from build123d import *

# Parameters (mm, degrees)
EXTRUDE_1_DEPTH     = 40
SKETCH_2_R          = 2
SKETCH_2_R_2        = 1.5
CUT_EXTRUDE_1_DEPTH = 112.803398875


with BuildPart() as part:
    # Эскиз1 → Бобышка-Вытянуть1 (new body)
    with BuildSketch(Plane.XY):
        with BuildLine():
            Line((0, 0), (100, 0))
            Line((100, 0), (100, 14))
            Line((100, 14), (84.933034374, 14))
            ThreePointArc((84.933034374, 14), (70, 15), (84.933034374, 16))
            Line((84.933034374, 16), (100, 16))
            Line((100, 16), (100, 30))
            Line((100, 30), (0, 30))
            Line((0, 30), (0, 16))
            Line((0, 16), (15.066965626, 16))
            ThreePointArc((15.066965626, 16), (30, 15), (15.066965626, 14))
            Line((15.066965626, 14), (0, 14))
            Line((0, 14), (0, 0))
        make_face()
    extrude(amount=EXTRUDE_1_DEPTH)

    # Эскиз2 → Вырез-Вытянуть1 (cut, through all)
    with BuildSketch(Plane.XZ):
        with Locations(Location((7.5, 30, 0), (0, 0, 270))):
            Circle(SKETCH_2_R)
        with Locations(Location((7.5, 10, 0), (0, 0, 270))):
            Circle(SKETCH_2_R)
        with Locations(Location((92.5, 30, 0), (0, 0, 270))):
            Circle(SKETCH_2_R)
        with Locations(Location((92.5, 10, 0), (0, 0, 270))):
            Circle(SKETCH_2_R)
        with Locations(Location((35, 32, 0), (0, 0, 270))):
            Circle(SKETCH_2_R_2)
        with Locations(Location((65, 32, 0), (0, 0, 270))):
            Circle(SKETCH_2_R_2)
        with Locations(Location((35, 8, 0), (0, 0, 270))):
            Circle(SKETCH_2_R_2)
        with Locations(Location((65, 8, 0), (0, 0, 270))):
            Circle(SKETCH_2_R_2)
    extrude(amount=-CUT_EXTRUDE_1_DEPTH, mode=Mode.SUBTRACT)


solid = part.part
The listing builds one solid part. Answer for the finished solid, in the listing's coordinates (mm). A direction names the side the tool comes from. Give positions to 0.01 mm unless a question says otherwise; leave off trailing zeros. Order: outer loops, then holes, each group sorted by start corner. A loop starts at its lowest first (then second) coordinate and runs counter-clockwise, first axis right, second up. Notation, with made-up numbers: (80.5, 84.5) - (107.5, 84.5) arc R14 ccw to (107.5, 108.5) - close; hole circle Ø5 at (71, 39.25). An arc over 180 degrees is marked (long way). Use one line per item in the form item = value.
1) Find section A-A on x = 22.5. Determine the outline of the cut face in (y, z).
Verdict:
outline = (0, 0) - (7.5, 0) - (7.5, 40) - (0, 40) - close; (22.5, 0) - (30, 0) - (30, 40) - (22.5, 40) - close
2) For faces 4 (the flat face through (92, 16, 20)), 5 (the flat face through (8, 14, 20)), 6 (the flat face through (49, 0, 20)), determine the directions among +Z, -Z, +X, -X, +Y, -Y from which every point of the face is accessible in a straight line to the end or side of a thin tool.
Verdict:
face_4 = +Z, -Z, +X
face_5 = +Z, -Z, -X
face_6 = +Z, -Z, +X, -X, -Y
3) Consider probe 1 along Y at (x, z) = (86, 34); probe 2 along X at (y, z) = (6.25, 10); probe 3 along X at (y, z) = (27, 29). Determine where each line is inside the solid, lowest interval first. Write a range as [from, to].
Verdict:
probe_1 = [0, 14], [16, 30]
probe_2 = [0, 5.5], [9.5, 90.5], [94.5, 100]
probe_3 = [0, 5.77], [9.23, 90.77], [94.23, 100]
4) Find section D-D on x = 7.5. Determine the outline of the cut face in (y, z), and give its area (3 significant figures).
Verdict:
outline = (0, 0) - (14, 0) - (14, 8) - (0, 8) - close; (0, 12) - (14, 12) - (14, 28) - (0, 28) - close; (0, 32) - (14, 32) - (14, 40) - (0, 40) - close; (16, 0) - (30, 0) - (30, 8) - (16, 8) - close; (16, 12) - (30, 12) - (30, 28) - (16, 28) - close; (16, 32) - (30, 32) - (30, 40) - (16, 40) - close
area = 896 mm^2
5) The mould has two halves that part along Z. Classify faces 1 (the cylindrical face through (94.483, 22.902, 10.26)), 2 (the flat face through (49, 15, 0)), 3 (the flat face through (100, 7, 20)): released by +Z, released by -Z, zero draft, split by the parting line, or undercut.
Verdict:
face_1 = undercut
face_2 = released by -Z
face_3 = zero draft
6) Find section B-B on x = 35. Determine the outline of the cut face in (y, z), and give its area (3 significant figures).
Verdict:
outline = (0, 0) - (30, 0) - (30, 6.5) - (0, 6.5) - close; (0, 9.5) - (30, 9.5) - (30, 30.5) - (0, 30.5) - close; (0, 33.5) - (30, 33.5) - (30, 40) - (0, 40) - close
area = 1,020 mm^2
7) Find section C-C on y = 8.75. Give the number of separate pieces and of enclosed holes in the cut face, and give its area (3 significant figures).
Verdict:
separate_pieces = 3
enclosed_holes = 8
area = 3,260 mm^2
